Check sheet for the modelled part. Datum: model origin and axes. Units: mm. A direction names the side the tool comes from. Coordinates: 2 decimals unless noted, no trailing zeros. Loops run counter-clockwise (first coordinate to the right, second up) from the corner with the lowest first, then second, coordinate; pieces in that order, holes last. Notation, with made-up numbers: (-27.75, 63) -> (-20.75, 63) arc R13 cw to (-20.75, 79) -> close; hole circle Ø7 at (73, 7.25). An arc over 180 degrees is marked (long way). Use CSV: the item, a comma, the result in double quotes.
```python
from build123d import *

# Parameters (mm, degrees)
SKETCH1_W           = 144
SKETCH1_H           = 125.68
BOSS_EXTRUDE1_DEPTH = 3
SKETCH2_W           = 144
SKETCH2_H           = 125.68
SKETCH2_W_2         = 137.62694519
SKETCH2_H_2         = 121.548177757
BOSS_EXTRUDE2_DEPTH = 86
SKETCH4_W           = 94.55727782
SKETCH4_H           = 37.953937335
CUT_EXTRUDE1_DEPTH  = 20
SKETCH6_W           = 39.790164022
SKETCH6_H           = 75.651590962
CUT_EXTRUDE3_DEPTH  = 20
SKETCH8_W           = 49.5692413
SKETCH8_H           = 91.849069086
BOSS_EXTRUDE3_DEPTH = 32
SKETCH7_W           = 45
SKETCH7_H           = 87.31
CUT_EXTRUDE4_DEPTH  = 32.17
SKETCH9_W           = 11.79717637
SKETCH9_H           = 31.86635219
CUT_EXTRUDE5_DEPTH  = 40
SKETCH10_W          = 11.687827299
SKETCH10_H          = 31.429738741
CUT_EXTRUDE6_DEPTH  = 40
SKETCH11_W          = 16.650134538
SKETCH11_H          = 74.314635754
SKETCH11_W_2        = 24.505886262
CUT_EXTRUDE7_DEPTH  = 40


with BuildPart() as part:
    # Sketch1 → Boss-Extrude1 (new body)
    with BuildSketch(Plane(origin=(0, 0, 0), x_dir=(1, 0, 0), z_dir=(0, 1, 0))):
        with Locations((-0.900426333, 18.508659662)):
            Rectangle(SKETCH1_W, SKETCH1_H)
    extrude(amount=BOSS_EXTRUDE1_DEPTH)

    # Sketch2 → Boss-Extrude2 (add)
    with BuildSketch(Plane(origin=(0, 3, 0), x_dir=(1, 0, 0), z_dir=(0, 1, 0))):
        with Locations((-0.900426333, 18.508659662)):
            Rectangle(SKETCH2_W, SKETCH2_H)
        with Locations((-2.339827632, 18.478566742)):
            Rectangle(SKETCH2_W_2, SKETCH2_H_2, mode=Mode.SUBTRACT)
    extrude(amount=BOSS_EXTRUDE2_DEPTH)

    # Sketch4 → Cut-Extrude1 (cut)
    with BuildSketch(Plane(origin=(71.099573667, 0, 0), x_dir=(0, 0, -1), z_dir=(1, 0, 0))):
        with Locations((17.672764627, 50.079604952)):
            Rectangle(SKETCH4_W, SKETCH4_H)
    extrude(amount=-CUT_EXTRUDE1_DEPTH, mode=Mode.SUBTRACT)

    # Sketch6 → Cut-Extrude3 (cut)
    with BuildSketch(Plane.ZY.offset(72.900426333)):
        with Locations((19.353212204, 44.793227562)):
            Rectangle(SKETCH6_W, SKETCH6_H)
    extrude(amount=-CUT_EXTRUDE3_DEPTH, mode=Mode.SUBTRACT)

    # Sketch8 → Boss-Extrude3 (add)
    with BuildSketch(Plane(origin=(0, 3, 0), x_dir=(1, 0, 0), z_dir=(0, 1, 0))):
        with Locations((5.315093732, 20.62475692)):
            Rectangle(SKETCH8_W, SKETCH8_H)
    extrude(amount=BOSS_EXTRUDE3_DEPTH)

    # Sketch7 → Cut-Extrude4 (cut)
    with BuildSketch(Plane.XZ):
        with Locations((5.233997278, -20.691377503)):
            Rectangle(SKETCH7_W, SKETCH7_H)
    extrude(amount=-CUT_EXTRUDE4_DEPTH, mode=Mode.SUBTRACT)

    # Sketch9 → Cut-Extrude5 (cut)
    with BuildSketch(Plane.XZ.offset(-32.17)):
        with Locations((-9.959298471, -44.905011983)):
            Rectangle(SKETCH9_W, SKETCH9_H)
    extrude(amount=-CUT_EXTRUDE5_DEPTH, mode=Mode.SUBTRACT)

    # Sketch10 → Cut-Extrude6 (cut)
    with BuildSketch(Plane.XZ.offset(-32.17)):
        with Locations((19.967671673, 4.341983418)):
            Rectangle(SKETCH10_W, SKETCH10_H)
    extrude(amount=-CUT_EXTRUDE6_DEPTH, mode=Mode.SUBTRACT)

    # Sketch11 → Cut-Extrude7 (cut)
    with BuildSketch(Plane.XZ):
        with Locations((50.891184892, -21.453909531)):
            Rectangle(SKETCH11_W, SKETCH11_H)
        with Locations((-43.781754887, -21.453909531)):
            Rectangle(SKETCH11_W_2, SKETCH11_H)
    extrude(amount=-CUT_EXTRUDE7_DEPTH, mode=Mode.SUBTRACT)


solid = part.part
```
1) Cross-section at D-D on y = 47.5. Record the boundary of the cut face in (x, z), and give its area (3 significant figures).
Answer below:
outline,"(-72.9, -81.35) -> (71.1, -81.35) -> (71.1, -64.95) -> (66.47, -64.95) -> (66.47, -79.25) -> (-71.15, -79.25) -> (-71.15, -0.54) -> (-72.9, -0.54) -> close; (-72.9, 39.25) -> (-71.15, 39.25) -> (-71.15, 42.3) -> (66.47, 42.3) -> (66.47, 29.61) -> (71.1, 29.61) -> (71.1, 44.33) -> (-72.9, 44.33) -> close"
area,"863 mm²"
2) Access from +Z, -Z, +X, -X, +Y, -Y to the whole of each face (thin tool, end or side, straight path). Record for faces 1 (the flat face through (-17.266, 16, -21)), 2 (the flat face through (-2, 44, 44.331)), 3 (the flat face through (66.474, 26, -18)), 4 (the flat face through (69, 50, 29.606)).
Answer below:
face 1,"-Y"
face 2,"+Z, +X, -X, +Y, -Y"
face 3,"+Y"
face 4,"+X, -X"
3) Cross-section at B-B on x = -14. Record the boundary of the cut face in (y, z), and give its area (3 significant figures).
Answer below:
outline,"(0, -81.35) -> (89, -81.35) -> (89, -79.25) -> (3, -79.25) -> (3, -66.55) -> (35, -66.55) -> (35, -60.84) -> (32.17, -60.84) -> (32.17, -64.35) -> (0, -64.35) -> close; (0, 22.96) -> (32.17, 22.96) -> (32.17, -28.97) -> (35, -28.97) -> (35, 25.3) -> (3, 25.3) -> (3, 42.3) -> (89, 42.3) -> (89, 44.33) -> (0, 44.33) -> close"
area,"773 mm²"
4) Thickness scan on line 1 along Z through (x, y) = (15.5, 26); line 2 along X through (y, z) = (28.5, -59); line 3 along Z through (x, y) = (58, 41). Record the ranges inside material, lowest first. Write a range as from..to.
Answer below:
line 1,"z = -81.35..-79.25, -66.55..-64.35, 22.96..25.3, 42.3..44.33"
line 2,"x = -72.9..-71.15, -19.47..-17.27, 27.73..30.1, 66.47..71.1"
line 3,"z = -81.35..-79.25, 42.3..44.33"
5) Cross-section at C-C on z = -37. Give the number of separate pieces and of enclosed holes in the cut face, and give its area (3 significant figures).
Answer below:
separate pieces,"5"
enclosed holes,"0"
area,"786 mm²"
6) Draft check along Y on faces 5 (the flat face through (-19.47, 19, -20)), 6 (the flat face through (69, 69.057, -17)), 7 (the flat face through (5, 32.17, -20)), 8 (the flat face through (69, 50, -64.951)). Enter one of: released by +Y, released by -Y, zero draft, split by the parting line, or undercut.
Answer below:
face 5,"zero draft"
face 6,"undercut"
face 7,"released by -Y"
face 8,"undercut"
7) Cross-section at A-A on y = 23. Record the boundary of the cut face in (x, z), and give its area (3 significant figures).
Answer below:
outline,"(-72.9, -81.35) -> (71.1, -81.35) -> (71.1, 44.33) -> (-72.9, 44.33) -> (-72.9, 39.25) -> (-71.15, 39.25) -> (-71.15, 42.3) -> (66.47, 42.3) -> (66.47, -79.25) -> (-71.15, -79.25) -> (-71.15, -0.54) -> (-72.9, -0.54) -> close; (-19.47, -66.55) -> (30.1, -66.55) -> (30.1, 25.3) -> (-19.47, 25.3) -> close; hole (-17.27, -64.35) -> (27.73, -64.35) -> (27.73, 22.96) -> (-17.27, 22.96) -> close"
area,"1,920 mm²"
8) Go/stop test with flat-tipped pins: pin 1 Ø6 at (x, z) = (-6.5, -10.5) entering from +Y; pin 2 Ø1.9 at (x, z) = (-71.5, 22.5) entering from -Y; pin 3 Ø5 at (x, z) = (1.5, 31) entering from +Y; pin 4 Ø1.4 at (y, z) = (33.5, -51) entering from +X. Record where each tip stops, or that it passes through.
Answer below:
pin 1,"stops at y = 35"
pin 2,"stops at y = 0"
pin 3,"stops at y = 3"
pin 4,"stops at x = 30.1"
